```python
from build123d import *

# Parameters (mm, degrees)
SKETCH1_R           = 8.001
SKETCH1_R_2         = 4.0005
BOSS_EXTRUDE1_DEPTH = 4.9784
SKETCH2_R           = 7.2898
SKETCH2_R_2         = 5.1435
CUT_EXTRUDE1_DEPTH  = 0.4572
SKETCH3_R           = 7.2898
SKETCH3_R_2         = 5.1435
CUT_EXTRUDE2_DEPTH  = 0.4572


with BuildPart() as part:
    # Sketch1 → Boss-Extrude1 (new body)
    with BuildSketch(Plane.XY):
        Circle(SKETCH1_R)
        Circle(SKETCH1_R_2, mode=Mode.SUBTRACT)
    extrude(amount=BOSS_EXTRUDE1_DEPTH)

    # Sketch2 → Cut-Extrude1 (cut)
    with BuildSketch(Plane.XY.offset(4.9784)):
        Circle(SKETCH2_R)
        Circle(SKETCH2_R_2, mode=Mode.SUBTRACT)
    extrude(amount=-CUT_EXTRUDE1_DEPTH, mode=Mode.SUBTRACT)

    # Sketch3 → Cut-Extrude2 (cut)
    with BuildSketch(Plane(origin=(0, 0, 0), x_dir=(-1, 0, 0), z_dir=(0, 0, -1))):
        Circle(SKETCH3_R)
        Circle(SKETCH3_R_2, mode=Mode.SUBTRACT)
    extrude(amount=-CUT_EXTRUDE2_DEPTH, mode=Mode.SUBTRACT)


solid = part.part
```
Design review of the part built by this model. Coordinates are the model's own, in mm. A direction names the side the tool comes from. Coordinates: 2 decimals unless noted, no trailing zeros. Write each loop counter-clockwise with the first axis right and the second up, starting at its lowest first coordinate (ties: lowest second). Pieces come first, ordered by that corner, then holes. Notation, with made-up numbers: M 5.5,17.25 L 37.5,17.25 A28 cw 37.5,53.25 Z; hole C 78.25,44.25 d3. An arc over 180 degrees is marked long. Answer as a JSON object with one key per item and string values.
Item 1: Insertion check: pin 1 Ø1 at (x, z) = (-3, 2.5) entering from -Y; pin 2 Ø2 at (x, z) = (-3.5, 0.5) entering from +Y; pin 3 Ø2 at (y, z) = (-4.5, 3) entering from +X. Each pin has a flat end and moves straight along its axis. Give the tip position at first contact, or say it passes through.
Outcome:
{"pin 1": "y = -7.6", "pin 2": "y = 7.6", "pin 3": "x = 7.19"}
Item 2: Add section A-A, the plane y = 0. Give the boundary of the cut face in (x, z).
Outcome:
{"outline": "M -8,0 L -7.29,0 L -7.29,0.46 L -5.14,0.46 L -5.14,0 L -4,0 L -4,4.98 L -5.14,4.98 L -5.14,4.52 L -7.29,4.52 L -7.29,4.98 L -8,4.98 Z; M 4,0 L 5.14,0 L 5.14,0.46 L 7.29,0.46 L 7.29,0 L 8,0 L 8,4.98 L 7.29,4.98 L 7.29,4.52 L 5.14,4.52 L 5.14,4.98 L 4,4.98 Z"}
Item 3: Wall thickness on probe 1 along Y at (x, z) = (0, 0.25); probe 2 along Y at (x, z) = (0, 3.75); probe 3 along Z at (x, y) = (1.75, 6.75): over which ranges is each line inside the solid? List them lowest first.
Outcome:
{"probe 1": "-8 to -7.29, -5.14 to -4, 4 to 5.14, 7.29 to 8", "probe 2": "-8 to -4, 4 to 8", "probe 3": "0.46 to 4.52"}
Item 4: Add section C-C, the plane z = 2.45. Give the boundary of the cut face in (x, y).
Outcome:
{"outline": "C 0,0 d16; hole C 0,0 d8"}
Item 5: Draft analysis for pull direction X (two halves, no side actions). For faces 4 (the cylindrical face through (-1.73, -7.81, 2.45)), 5 (the cylindrical face through (0.67, 5.1, 0.23)), 6 (the flat face through (2.3, -7.1, 4.978)), 7 (the cylindrical face through (-5.78, -4.44, 4.75)), state which applies: pulls with the +X half, pulls with the -X half, needs draft (parallel to the pull), parting line crosses it, or undercut.
Outcome:
{"face 4": "parting line crosses it", "face 5": "undercut", "face 6": "needs draft", "face 7": "undercut"}
Item 6: Add section D-D, the plane y = -5.5. Give the boundary of the cut face in (x, z).
Outcome:
{"outline": "M -5.81,0 L -4.78,0 L -4.78,0.46 L 4.78,0.46 L 4.78,0 L 5.81,0 L 5.81,4.98 L 4.78,4.98 L 4.78,4.52 L -4.78,4.52 L -4.78,4.98 L -5.81,4.98 Z"}
Item 7: Machinability: for faces 1 (the flat face through (5, -2, 0.457)), 2 (the flat face through (-5, -2, 4.521)), 3 (the cylindrical face through (-0.9, -3.9, 2.5)), which of the approach directions +Z, -Z, +X, -X, +Y, -Y give a long, thin tool a straight path to every point of the face, cutting with its end or side? Answer none if there is none.
Outcome:
{"face 1": "-Z", "face 2": "+Z", "face 3": "+Z, -Z"}
